The figure shows three views and two pictorial views of one solid part (mm, origin at its lowest corner). Answer the questions. Give positions to 0.01 mm unless a question says otherwise; leave off trailing zeros. Write each loop counter-clockwise with the first axis right and the second up, starting at its lowest first coordinate (ties: lowest second). Pieces come first, ordered by that corner, then holes. Notation, with made-up numbers: (26.25, -32.75) - (56.25, -32.75) arc R26 cw to (56.25, -17.75) - close; hole circle Ø11 at (2.5, 69.25). An arc over 180 degrees is marked (long way). Use CSV: the item, a comma, the result in double quotes. Start each with the question number.
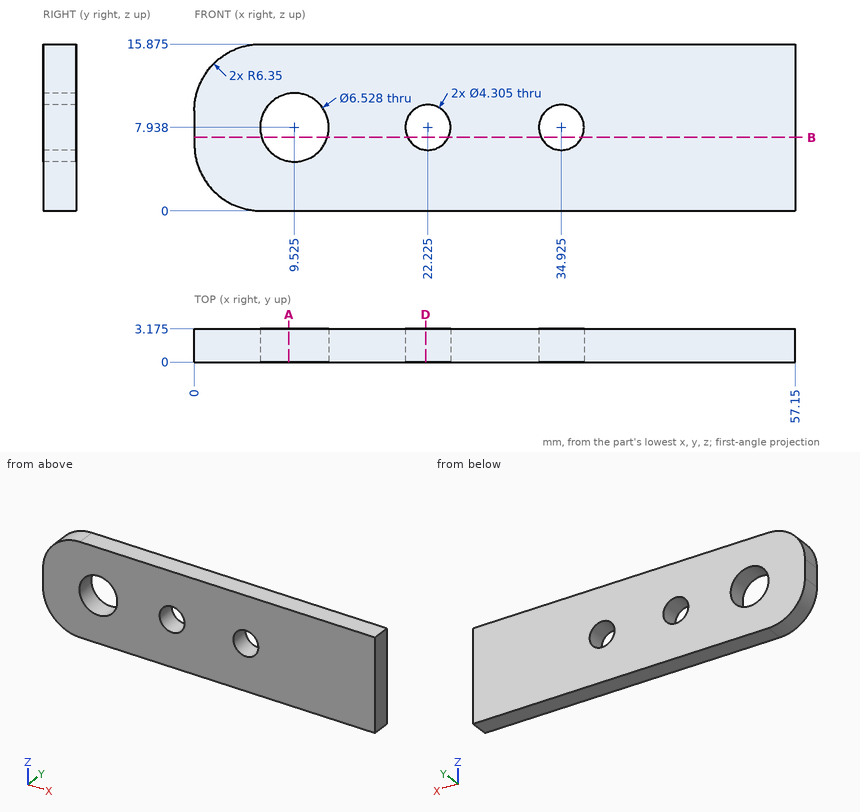
(1) Given P1, Ø3.5, axis at x = 34.93, z = 7.94, coming from the +Y side, flat-ended and moving along its own axis, determine where the tip first touches the part or whether it passes through.
(2) The part is cut by section B-B on z = 7. Give the number of separate pieces and of enclosed holes in the cut face, plus the area to 3 significant figures.
(3) Consider probe 1 along X at (y, z) = (0.9, 8); probe 2 along Z at (x, y) = (22.5, 2.9) (1 decimal); probe 3 along X at (y, z) = (2, 10.25). Determine where each line is inside the solid, lowest interval first.
(4) The part is cut by section A-A on x = 9. Write down the section's boundary in (y, z) (1 decimal).
(5) The part is cut by section D-D on x = 22. Write down the section's boundary in (y, z) (1 decimal).
Reported:
1,P1,"through"
2,separate pieces,"4"
2,enclosed holes,"0"
2,area,"137 mm²"
3,probe 1,"0 to 6.26, 12.79 to 20.07, 24.38 to 32.77, 37.08 to 57.15"
3,probe 2,"0 to 5.8, 10.1 to 15.9"
3,probe 3,"0.04 to 7.22, 11.83 to 57.15"
4,outline,"(0, 0) - (3.2, 0) - (3.2, 4.7) - (0, 4.7) - close; (0, 11.2) - (3.2, 11.2) - (3.2, 15.9) - (0, 15.9) - close"
5,outline,"(0, 0) - (3.2, 0) - (3.2, 5.8) - (0, 5.8) - close; (0, 10.1) - (3.2, 10.1) - (3.2, 15.9) - (0, 15.9) - close"
